```python
from build123d import *

# Parameters (mm, degrees)
CUT_EXTRUDE4_DEPTH      = 5
CROQUIS1_R              = 1.25
SALIENTE_EXTRUIR1_DEPTH = 3
CROQUIS2_R              = 5
CROQUIS2_R_2            = 3.875
CORTAR_EXTRUIR2_DEPTH   = 5


with BuildPart() as part:
    # Sketch1 → Revolve1 (revolve)
    with BuildSketch(Plane.XY):
        with BuildLine():
            Line((4.304738622, -13), (4.304738622, -16.832856763))
            Line((4.304738622, -16.832856763), (3.137595386, -18))
            Line((3.137595386, -18), (0, -18))
            Line((0, -18), (0, -13))
            Line((0, -13), (0, 0))
            Line((0, 0), (0, 5.5))
            Line((0, 5.5), (3.464101615, 5.5))
            ThreePointArc((3.464101615, 5.5), (6.492002013, 0.322350532), (3.991907406, -5.129783159))
            ThreePointArc((3.991907406, -5.129783159), (2.699987373, -8.799256044), (5.5, -11.5))
            Line((5.5, -11.5), (6.5, -11.5))
            Line((6.5, -11.5), (6.5, -13))
            Line((6.5, -13), (4.304738622, -13))
        make_face()
    revolve(axis=Axis((0, -13, 0), (0, 1, 0)))

    # Sketch5 → Cut-Extrude4 (cut)
    with BuildSketch(Plane.XZ.offset(13)):
        with BuildLine():
            Line((-5, 4.153311931), (-5, -4.153311931))
            ThreePointArc((-5, -4.153311931), (-6.5, 0), (-5, 4.153311931))
        make_face()
        with BuildLine():
            Line((5, -4.153311931), (5, 4.153311931))
            ThreePointArc((5, 4.153311931), (6.5, 0), (5, -4.153311931))
        make_face()
    extrude(amount=-CUT_EXTRUDE4_DEPTH, mode=Mode.SUBTRACT)

    # Croquis1 → Saliente-Extruir1 (add)
    with BuildSketch(Plane(origin=(0, -18, 0), x_dir=(-1, 0, 0), z_dir=(0, -1, 0))):
        Circle(CROQUIS1_R)
    extrude(amount=SALIENTE_EXTRUIR1_DEPTH)

    # Croquis2 → Cortar-Extruir2 (cut)
    with BuildSketch(Plane.XZ.offset(18)):
        Circle(CROQUIS2_R)
        Circle(CROQUIS2_R_2, mode=Mode.SUBTRACT)
    extrude(amount=-CORTAR_EXTRUIR2_DEPTH, mode=Mode.SUBTRACT)


solid = part.part
```
Geometry check sheet. Reference: the model listing, model coordinates, mm. A direction names the side the tool comes from. Coordinates: 2 decimals unless noted, no trailing zeros. Order: outer loops, then holes, each group sorted by start corner. A loop starts at its lowest first (then second) coordinate and runs counter-clockwise, first axis right, second up.
Q1. Tool access check on faces 4 (the face through (-0.504, -15.161, 3.842)), 5 (the face through (0, -11.5, -6)), 6 (the face through (5, -12, 0)). Record the directions out of +Z, -Z, +X, -X, +Y, -Y that give a thin tool (end or side, any length) a straight path to the whole face; none if there is none.
Reply:
face 4: -Y
face 5: -Z
face 6: +Z, -Z, +X, -Y
Q2. Sectioned sample at A-A on x = 0. Record the cut outline in (y, z) (3 decimals), and give its area (3 significant figures).
Reply:
outline: (-21, -1.25) - (-18, -1.25) - (-18, -3.138) - (-17.263, -3.875) - (-13, -3.875) - (-13, -6.5) - (-11.5, -6.5) - (-11.5, -5.5) arc R3.599 cw to (-5.13, -3.992) arc R6.5 ccw to (5.5, -3.464) - (5.5, 3.464) arc R6.5 ccw to (-5.13, 3.992) arc R3.599 cw to (-11.5, 5.5) - (-11.5, 6.5) - (-13, 6.5) - (-13, 3.875) - (-17.263, 3.875) - (-18, 3.138) - (-18, 1.25) - (-21, 1.25) - close
area: 226 mm2
Q3. Sectioned sample at B-B on y = 1.75. Record the cut outline in (x, z).
Reply:
outline: circle Ø12.52 at (0, 0)
Q4. Thickness scan on probe 1 along Y at (x, z) = (4.5, -1.5); probe 2 along Y at (x, z) = (-3.75, 0.25); probe 3 along Y at (x, z) = (-0.5, -2). Record the ranges inside material, lowest first.
Reply:
probe 1: y = -13 to -11.26, -4.44 to 4.44
probe 2: y = -17.38 to -10.61, -5.33 to 5.3
probe 3: y = -18 to 5.5
Q5. Depth check by flat-ended pin: pin 1 Ø0.8 at (y, z) = (-12.5, 1.5) entering from +X; pin 2 Ø3.5 at (x, z) = (-0.5, -5.5) entering from +Y; pin 3 Ø1.5 at (x, y) = (-4.5, -3.5) entering from +Z. Enter the tip coordinate at first touch or a pass-through.
Reply:
pin 1: stops at x = 5
pin 2: stops at y = 5.29
pin 3: stops at z = 4.21
Q6. Draft check along Y on faces 1 (the face through (1, -18, 1)), 2 (the face through (0, -11.5, 6)), 3 (the face through (-0.1, -12.3, 6.5)). Enter one of: released by +Y, released by -Y, zero draft, split by the parting line, or undercut.
Reply:
face 1: released by -Y
face 2: undercut
face 3: zero draft
Q7. Sectioned sample at C-C on z = 0. Record the cut outline in (x, y) (3 decimals).
Reply:
outline: (-5, -13) - (-3.875, -13) - (-3.875, -17.263) - (-3.138, -18) - (-1.25, -18) - (-1.25, -21) - (1.25, -21) - (1.25, -18) - (3.138, -18) - (3.875, -17.263) - (3.875, -13) - (5, -13) - (5, -11.362) arc R3.599 cw to (3.992, -5.13) arc R6.5 ccw to (3.464, 5.5) - (-3.464, 5.5) arc R6.5 ccw to (-3.992, -5.13) arc R3.599 cw to (-5, -11.362) - close
